```python
from build123d import *

# Parameters (mm, degrees)
SKETCH4_R          = 1.65
CUT_EXTRUDE1_DEPTH = 4
CUT_EXTRUDE2_START = 4
SKETCH5_R          = 2.9
CUT_EXTRUDE2_DEPTH = 15
SKETCH7_R          = 6.5
CUT_EXTRUDE4_DEPTH = 10
SKETCH10_R         = 1.65
CUT_EXTRUDE5_DEPTH = 6
CUT_EXTRUDE6_START = -1.7
CUT_EXTRUDE6_DEPTH = 2.6


with BuildPart() as part:
    # Sketch1 → Revolve1 (revolve)
    with BuildSketch(Plane.XY):
        Polygon((0, 0), (63, 0), (69, 10), (0, 10), align=None)
    revolve(axis=Axis((0, 10, 0), (0, -1, 0)))

    # Sketch4 → Cut-Extrude1 (cut)
    with BuildSketch(Plane(origin=(0, 0, 0), x_dir=(1, 0, 0), z_dir=(0, 1, 0))):
        with Locations((34.749254443, 17.70562949)):
            Circle(SKETCH4_R)
        with Locations((51.602562721, 28.603767595)):
            Circle(SKETCH4_R)
        with Locations((51.602562721, -28.603767595)):
            Circle(SKETCH4_R)
        with Locations((34.749254443, -17.70562949)):
            Circle(SKETCH4_R)
        with Locations((-34.749254443, -17.70562949)):
            Circle(SKETCH4_R)
        with Locations((-51.602562721, -28.603767595)):
            Circle(SKETCH4_R)
        with Locations((-51.602562721, 28.603767595)):
            Circle(SKETCH4_R)
        with Locations((-34.749254443, 17.70562949)):
            Circle(SKETCH4_R)
    extrude(amount=CUT_EXTRUDE1_DEPTH, mode=Mode.SUBTRACT)

    # Sketch5 → Cut-Extrude2 (cut, through all)
    with BuildSketch(Plane(origin=(0, 0, 0), x_dir=(-1, 0, 0), z_dir=(0, -1, 0)).offset(CUT_EXTRUDE2_START)):
        with Locations((-51.602562721, 28.603767595)):
            Circle(SKETCH5_R)
        with Locations((-51.602562721, -28.603767595)):
            Circle(SKETCH5_R)
        with Locations((51.602562721, -28.603767595)):
            Circle(SKETCH5_R)
        with Locations((51.602562721, 28.603767595)):
            Circle(SKETCH5_R)
        with Locations((-34.749254443, 17.70562949)):
            Circle(SKETCH5_R)
        with Locations((-34.749254443, -17.70562949)):
            Circle(SKETCH5_R)
        with Locations((34.749254443, -17.70562949)):
            Circle(SKETCH5_R)
        with Locations((34.749254443, 17.70562949)):
            Circle(SKETCH5_R)
    extrude(amount=-CUT_EXTRUDE2_DEPTH, mode=Mode.SUBTRACT)

    # Sketch7 → Cut-Extrude4 (cut)
    with BuildSketch(Plane(origin=(0, 0, 0), x_dir=(-1, 0, 0), z_dir=(0, -1, 0))):
        with Locations((-15.39090645, 42.286167935)):
            Circle(SKETCH7_R)
    extrude(amount=-CUT_EXTRUDE4_DEPTH, mode=Mode.SUBTRACT)

    # Sketch10 → Cut-Extrude5 (cut)
    with BuildSketch(Plane(origin=(0, 10, 0), x_dir=(-1, 0, 0), z_dir=(0, 1, 0))):
        with Locations((-8, 56)):
            Circle(SKETCH10_R)
        with Locations((8, 56)):
            Circle(SKETCH10_R)
        with Locations((8, 24)):
            Circle(SKETCH10_R)
        with Locations((-8, 24)):
            Circle(SKETCH10_R)
        with BuildLine():
            Line((-13, 32.25), (7, 32.25))
            Line((7, 32.25), (7, 47.75))
            Line((7, 47.75), (-23, 47.75))
            ThreePointArc((-23, 47.75), (-29.960784303, 44.455040042), (-31.824789595, 36.982773752))
            Line((-31.824789595, 36.982773752), (-28.486695571, 20.31372674))
            ThreePointArc((-28.486695571, 20.31372674), (-28.121971433, 17.871279613), (-28, 15.40476494))
            Line((-28, 15.40476494), (-28, -13))
            ThreePointArc((-28, -13), (-26.535533906, -16.535533906), (-23, -18))
            Line((-23, -18), (23, -18))
            ThreePointArc((23, -18), (26.535533906, -16.535533906), (28, -13))
            Line((28, -13), (28, 13))
            ThreePointArc((28, 13), (26.535533906, 16.535533906), (23, 18))
            Line((23, 18), (-9, 18))
            ThreePointArc((-9, 18), (-11.828427125, 19.171572875), (-13, 22))
            Line((-13, 22), (-13, 32.25))
        make_face()
    extrude(amount=-CUT_EXTRUDE5_DEPTH, mode=Mode.SUBTRACT)

    # Sketch11 → Cut-Extrude6 (cut)
    with BuildSketch(Plane(origin=(0, 10, 0), x_dir=(-1, 0, 0), z_dir=(0, 1, 0)).offset(CUT_EXTRUDE6_START)):
        Polygon((-4.651368439, 56), (-6.325684219, 58.9), (-9.674315781, 58.9), (-11.348631561, 56), (-9.674315781, 53.1), (-6.325684219, 53.1), align=None)
        Polygon((11.347570698, 56.084283782), (9.600793452, 58.941223157), (6.253222754, 58.856939374), (4.652429302, 55.915716218), (6.399206548, 53.058776843), (9.746777246, 53.143060626), align=None)
        Polygon((-5.1, 25.674315781), (-8, 27.348631561), (-10.9, 25.674315781), (-10.9, 22.325684219), (-8, 20.651368439), (-5.1, 22.325684219), align=None)
        Polygon((10.898923771, 22.323821518), (10.901075032, 25.672452388), (8.002151261, 27.34863087), (5.101076229, 25.676178482), (5.098924968, 22.327547612), (7.997848739, 20.65136913), align=None)
    extrude(amount=-CUT_EXTRUDE6_DEPTH, mode=Mode.SUBTRACT)


solid = part.part
```
Geometry: final body of the model. Coordinates: model frame, mm. A direction names the side the tool comes from. Coordinates: 2 decimals unless noted, no trailing zeros. Order: outer loops, then holes, each group sorted by start corner. A loop starts at its lowest first (then second) coordinate and runs counter-clockwise, first axis right, second up.
Item 1: Section query B-B (z = 0). Output: boundary loops of the cut face in (x, y), then the cut area to 3 significant figures.
Answer:
outline: (-69, 10) - (-63, 0) - (63, 0) - (69, 10) - (28, 10) - (28, 4) - (-28, 4) - (-28, 10) - close
area: 984 mm2
Item 2: Access query for faces 1 (the face through (-6.7, 8.3, 22.6)), 2 (the face through (-1, 10, -30)), 3 (the face through (8, 4, 24)). Directions: +Z, -Z, +X, -X, +Y, -Y. A direction counts if a zero-diameter tool reaches every point of the face in a straight line with its end or side. Return the directions, or none.
Answer:
face 1: none
face 2: +Z, -Z, +X, -X, +Y
face 3: +Y
Item 3: Draft query along Z for faces 4 (the face through (16.24, 4.93, -48.73)), 5 (the face through (1, 0, 1)), 6 (the face through (-13.74, 0.63, -61.87)), 7 (the face through (13, 7, 27)). Return one class per face: released by +Z, released by -Z, zero draft, split by the parting line, or undercut.
Answer:
face 4: undercut
face 5: zero draft
face 6: split by the parting line
face 7: undercut
Item 4: Contact query for flat-ended pins moving along their axis: P1, Ø2, axis at x = 2.5, y = 1.5, coming from the -Z side; P2, Ø1.8, axis at y = 6.5, z = 6.5, coming from the +X side; P3, Ø1.3, axis at y = 7, z = 24, coming from the +X side; P4, Ø4.5, axis at x = -51.6, z = 28.6, coming from the +Y side. Output: stop coordinate, or through.
Answer:
P1: stops at z = -64.45
P2: stops at x = 67.13
P3: stops at x = 63.25
P4: passes through
Item 5: Section query C-C (y = 2.5). State how many separate pieces and enclosed holes the cut face has, then the cut area to 3 significant figures.
Answer:
separate pieces: 1
enclosed holes: 9
area: 12,700 mm2
Item 6: Section query A-A (x = 0). Output: boundary loops of the cut face in (y, z).
Answer:
outline: (0, -63) - (10, -69) - (10, -18) - (4, -18) - (4, 18) - (10, 18) - (10, 32.25) - (4, 32.25) - (4, 47.75) - (10, 47.75) - (10, 69) - (0, 63) - close
Item 7: Material intervals for line 1 along X through (y, z) = (3, -31); line 2 along Z through (x, y) = (-8, 7.5); line 3 along Z through (x, y) = (-8, 4.6), sorted ascending.
Answer:
line 1: x = -56.9 to -53.24, -49.97 to 49.97, 53.24 to 56.9
line 2: z = -67.02 to -18, 18 to 20.65, 27.35 to 53.1, 58.9 to 67.02
line 3: z = -65.27 to -18, 18 to 22.35, 25.65 to 54.35, 57.65 to 65.27
